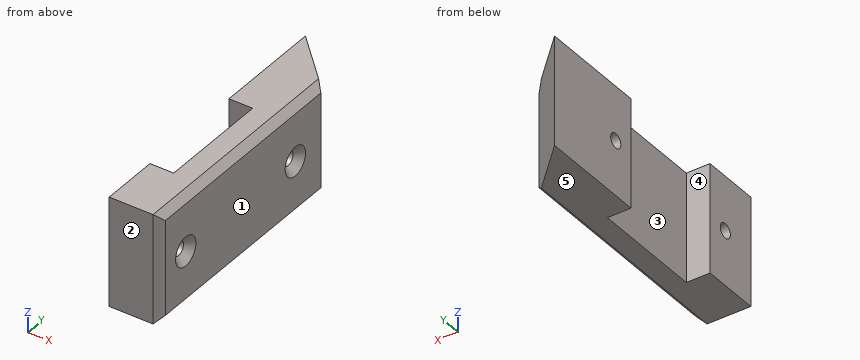
```python
from build123d import *

# Parameters (mm, degrees)
PAD_DEPTH       = 7.5
SKETCH001_R     = 1
POCKET_DEPTH    = 7.001
CHAMFER_SIZE    = 1
CHAMFER001_SIZE = 1


with BuildPart() as part:
    # Sketch → Pad (new body, symmetric)
    with BuildSketch(Plane.XY):
        Polygon((0, 0), (0, -15), (3.25, -15), (3.25, -30.5), (0, -30.5), (0, -38.5), (7, -38.5), (7, -7), align=None)
    extrude(amount=PAD_DEPTH, both=True)

    # Sketch001 (on Face7 of Pad) → Pocket (cut, through all)
    with BuildSketch(Plane.YZ.offset(7)):
        with Locations((-33.5, 0)):
            Circle(SKETCH001_R)
        with Locations((-12, 0)):
            Circle(SKETCH001_R)
    extrude(amount=-POCKET_DEPTH, mode=Mode.SUBTRACT)

    # Chamfer
    chamfer_edges = [part.edges().sort_by_distance(p)[0] for p in [
        (7, -13, 0),
        (7, -34.5, 0),
    ]]
    chamfer(chamfer_edges, length=CHAMFER_SIZE)

    # Chamfer001
    chamfer001_edges = [part.edges().sort_by_distance(p)[0] for p in [
        (7, -22.75, 7.5),
        (7, -38.5, 0),
        (7, -22.75, -7.5),
    ]]
    chamfer(chamfer001_edges, length=CHAMFER001_SIZE)


solid = part.part
```
The listing builds one solid part. Answer for the finished solid, in the listing's coordinates (mm). Face numbers are marked on the shaded views. A direction names the side the tool comes from. Give positions to 0.01 mm unless a question says otherwise; leave off trailing zeros. Order: outer loops, then holes, each group sorted by start corner. A loop starts at its lowest first (then second) coordinate and runs counter-clockwise, first axis right, second up. Notation, with made-up numbers: (-39.5, 36.25) -> (8.5, 36.25) arc R10 cw to (8.5, 48.25) -> close; hole circle Ø6 at (43, 28.5). An arc over 180 degrees is marked (long way). Answer as a JSON object with one key per item and string values. Group by question number.
Item 1: The part is cut by section C-C on y = -33.5. Write down the section's boundary in (x, z).
Item 2: The part is cut by section B-B on z = 0. Write down the section's boundary in (x, y).
Item 3: A tool of negligible diameter and unlimited length cuts with its end or side. For the marked faces 4 and 5, from which of +Z, -Z, +X, -X, +Y, -Y can it reach the whole face along a straight path? Write none if from no direction.
Item 4: The part is cut by section A-A on x = 2.5. Write down the section's boundary in (y, z).
Item 5: The part is cut by section D-D on x = 4.25. Write down the section's boundary in (y, z).
Item 6: Flat-ended cylindrical pins translate along their axes: pin 1 (3.5 mm diameter, centred on x = 1.5, z = 3.5, fed in from +Y); pin 2 (4 mm diameter, centred on y = -25, z = 0, fed in from -X). Find the tip coordinate at first contact, or state that the pin passes through.
Item 7: Consider L1, parallel to Z at x = 2.25, y = -33.5; L2, parallel to Y at x = 4.5, z = -0.25; L3, parallel to X at y = -9, z = -7. Determine where each line is inside the solid, lowest interval first. Write a range as from..to.
Item 8: Determine the mould class of the marked faces 1, 2 and 3 for opening direction Y: pulls with the +Y half, pulls with the -Y half, needs draft (parallel to the pull), parting line crosses it, or undercut.
Result set:
{
 "1": {"outline": "(0, -7.5) -> (6, -7.5) -> (7, -6.5) -> (7, -2) -> (6, -1) -> (0, -1) -> close; (0, 1) -> (6, 1) -> (7, 2) -> (7, 6.5) -> (6, 7.5) -> (0, 7.5) -> close"},
 "2": {"outline": "(0, -38.5) -> (6, -38.5) -> (7, -37.5) -> (7, -35.5) -> (6, -34.5) -> (0, -34.5) -> close; (0, -32.5) -> (6, -32.5) -> (7, -31.5) -> (7, -14) -> (6, -13) -> (0, -13) -> (0, -15) -> (3.25, -15) -> (3.25, -30.5) -> (0, -30.5) -> close; (0, -11) -> (6, -11) -> (7, -10) -> (7, -7) -> (0, 0) -> close"},
 "3": {"face 4": "+Z, -Z, -X", "face 5": "-Z, +X, -X, +Y, -Y"},
 "4": {"outline": "(-38.5, -7.5) -> (-30.5, -7.5) -> (-30.5, 7.5) -> (-38.5, 7.5) -> close; (-15, -7.5) -> (-2.5, -7.5) -> (-2.5, 7.5) -> (-15, 7.5) -> close; hole circle Ø2 at (-33.5, 0); hole circle Ø2 at (-12, 0)"},
 "5": {"outline": "(-38.5, -7.5) -> (-4.25, -7.5) -> (-4.25, 7.5) -> (-38.5, 7.5) -> close; hole circle Ø2 at (-33.5, 0); hole circle Ø2 at (-12, 0)"},
 "6": {"pin 1": "y = 0", "pin 2": "x = 3.25"},
 "7": {"L1": "-7.5..-1, 1..7.5", "L2": "-38.5..-34.47, -32.53..-12.97, -11.03..-4.5", "L3": "0..6.5"},
 "8": {"face 1": "needs draft", "face 2": "pulls with the -Y half", "face 3": "undercut"}
}
